Autodesk Inventor part; units mm, degrees
ref_plane "YZ Plane" through (0, 0, 0) normal (1, 0, 0) x (0, 1, 0)
ref_plane "XZ Plane" through (0, 0, 0) normal (0, 1, 0) x (-1, 0, 0)
sketch "Sketch1" plane through (0, 0, 0) normal (0, 0, 1) x (1, 0, 0)
  line L0 (0, 0) -> (9.3116, 0)
  line L1 (9.3116, 0) -> (9.3116, 7.8058)
  line L2 (9.3116, 7.8058) -> (0, 7.8058)
  line L3 (0, 7.8058) -> (0, 0)
  circle A0 centre (2.6618, 3.222) radius 0.7712
  dimension "d0" = 9.3116
  dimension "d1" = 7.8058
  dimension "d2" = 2.6618
  dimension "d3" = 3.222
  dimension "d4" = 1.5424
extrude "Extrusion1" add sketch "Sketch1" along normal blind 4
properties part number "testdelete"
Could you check a few things on this model? Use its own coordinates, in mm. Give positions to 0.01 mm unless a question says otherwise; leave off trailing zeros. Loops run counter-clockwise (first coordinate to the right, second up) from the corner with the lowest first, then second, coordinate; pieces in that order, holes last. Notation, with made-up numbers: (12.25, -37) - (54.25, -37) arc R24 cw to (54.25, -10) - close; hole circle Ø10 at (-11.75, -35). An arc over 180 degrees is marked (long way). Answer in a Markdown table with one row per item. Add a question column.
Q1. Please list where these lines run through material, in increasing order: L1, parallel to Y at x = 3.25, z = 1.8; L2, parallel to Y at x = 2.25, z = 1.65. Write a range as from..to.
Q2. If we section it at C-C (z = 2.1): List the corners of the cut face in (x, y) for me, plus the area to 3 significant figures.
Q3. If we section it at A-A (y = 3.75): List the corners of the cut face in (x, z) for me, plus the area to 3 significant figures.
Q4. We'd pull the mould along X, two halves only. Please class faces 1 (the face through (9.312, 4, 2)), 2 (the face through (5, 0, 2)), 3 (the face through (0, 4, 2)), 4 (the face through (3.018, 3.906, 1.972)): +X half, -X half, draft (parallel to the pull), parting line (faces both ways), or undercut.
Q5. If we section it at B-B (x = 3.25): List the corners of the cut face in (y, z) for me, plus the area to 3 significant figures.
The answers:
| question | item | result |
|---|---|---|
| 1 | L1 | y = 0..2.72, 3.72..7.81 |
| 1 | L2 | y = 0..2.57, 3.87..7.81 |
| 2 | outline | (0, 0) - (9.31, 0) - (9.31, 7.81) - (0, 7.81) - close; hole circle Ø1.54 at (2.66, 3.22) |
| 2 | area | 70.8 mm^2 |
| 3 | outline | (0, 0) - (2.1, 0) - (2.1, 4) - (0, 4) - close; (3.22, 0) - (9.31, 0) - (9.31, 4) - (3.22, 4) - close |
| 3 | area | 32.7 mm^2 |
| 4 | face 1 | +X half |
| 4 | face 2 | draft |
| 4 | face 3 | -X half |
| 4 | face 4 | undercut |
| 5 | outline | (0, 0) - (2.72, 0) - (2.72, 4) - (0, 4) - close; (3.72, 0) - (7.81, 0) - (7.81, 4) - (3.72, 4) - close |
| 5 | area | 27.2 mm^2 |
